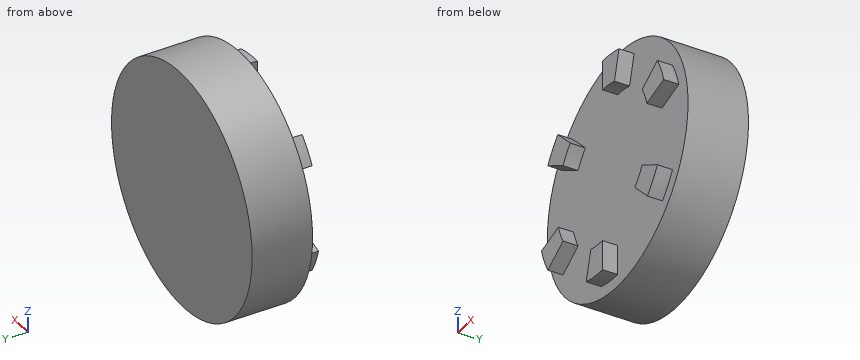
from build123d import *

# Parameters (mm, degrees)
F0_R     = 25.4
F1_DEPTH = 12.7
F2_DEPTH = 15.875


# Not quite as in the source:
# - a length typed as a fraction of an inch, garbled in the dataset ("3 / 203.2 mm" for 3/8 in), is restored
# - a feature names something its author has since deleted; it is built from what else it names


with BuildPart() as f1:
    # F0 (on Front) → F1 (new body)
    with BuildSketch(Plane.XZ):
        Circle(F0_R)
        with BuildLine():
            Line((0, -16.51), (0, -22.86))
            ThreePointArc((0, -22.86), (-2.9838287542, -22.664429531), (-5.916603371, -22.081064389))
            Line((-5.916603371, -22.081064389), (-4.2731024346, -15.947435392))
            ThreePointArc((-4.2731024346, -15.947435392), (-2.1549874336, -16.3687546613), (0, -16.51))
        make_face(mode=Mode.SUBTRACT)
        with BuildLine():
            Line((-14.2980794165, -8.255), (-19.7973407305, -11.43))
            ThreePointArc((-19.7973407305, -11.43), (-21.1198861132, -8.7481432639), (-22.081064389, -5.916603371))
            Line((-22.081064389, -5.916603371), (-15.947435392, -4.2731024346))
            ThreePointArc((-15.947435392, -4.2731024346), (-15.2532510818, -6.3181034683), (-14.2980794165, -8.255))
        make_face(mode=Mode.SUBTRACT)
        with BuildLine():
            Line((14.2980794165, -8.255), (19.7973407305, -11.43))
            ThreePointArc((19.7973407305, -11.43), (18.1360573591, -13.9162862671), (16.1644610179, -16.1644610179))
            Line((16.1644610179, -16.1644610179), (11.6743329574, -11.6743329574))
            ThreePointArc((11.6743329574, -11.6743329574), (13.0982636482, -10.0506511929), (14.2980794165, -8.255))
        make_face(mode=Mode.SUBTRACT)
        with BuildLine():
            Line((-14.2980794165, 8.255), (-19.7973407305, 11.43))
            ThreePointArc((-19.7973407305, 11.43), (-18.1360573591, 13.9162862671), (-16.1644610179, 16.1644610179))
            Line((-16.1644610179, 16.1644610179), (-11.6743329574, 11.6743329574))
            ThreePointArc((-11.6743329574, 11.6743329574), (-13.0982636482, 10.0506511929), (-14.2980794165, 8.255))
        make_face(mode=Mode.SUBTRACT)
        with BuildLine():
            Line((14.2980794165, 8.255), (19.7973407305, 11.43))
            ThreePointArc((19.7973407305, 11.43), (21.1198861132, 8.7481432639), (22.081064389, 5.916603371))
            Line((22.081064389, 5.916603371), (15.947435392, 4.2731024346))
            ThreePointArc((15.947435392, 4.2731024346), (15.2532510818, 6.3181034683), (14.2980794165, 8.255))
        make_face(mode=Mode.SUBTRACT)
        with BuildLine():
            Line((0, 16.51), (0, 22.86))
            ThreePointArc((0, 22.86), (2.9838287542, 22.664429531), (5.916603371, 22.081064389))
            Line((5.916603371, 22.081064389), (4.2731024346, 15.947435392))
            ThreePointArc((4.2731024346, 15.947435392), (2.1549874336, 16.3687546613), (0, 16.51))
        make_face(mode=Mode.SUBTRACT)
        with BuildLine():
            ThreePointArc((5.916603371, 22.081064389), (2.9838287542, 22.664429531), (0, 22.86))
            Line((0, 22.86), (0, 16.51))
            ThreePointArc((0, 16.51), (2.1549874336, 16.3687546613), (4.2731024346, 15.947435392))
            Line((4.2731024346, 15.947435392), (5.916603371, 22.081064389))
        make_face()
        with BuildLine():
            ThreePointArc((-16.1644610179, 16.1644610179), (-18.1360573591, 13.9162862671), (-19.7973407305, 11.43))
            Line((-19.7973407305, 11.43), (-14.2980794165, 8.255))
            ThreePointArc((-14.2980794165, 8.255), (-13.0982636482, 10.0506511929), (-11.6743329574, 11.6743329574))
            Line((-11.6743329574, 11.6743329574), (-16.1644610179, 16.1644610179))
        make_face()
        with BuildLine():
            ThreePointArc((-22.081064389, -5.916603371), (-21.1198861132, -8.7481432639), (-19.7973407305, -11.43))
            Line((-19.7973407305, -11.43), (-14.2980794165, -8.255))
            ThreePointArc((-14.2980794165, -8.255), (-15.2532510818, -6.3181034683), (-15.947435392, -4.2731024346))
            Line((-15.947435392, -4.2731024346), (-22.081064389, -5.916603371))
        make_face()
        with BuildLine():
            ThreePointArc((16.1644610179, -16.1644610179), (18.1360573591, -13.9162862671), (19.7973407305, -11.43))
            Line((19.7973407305, -11.43), (14.2980794165, -8.255))
            ThreePointArc((14.2980794165, -8.255), (13.0982636482, -10.0506511929), (11.6743329574, -11.6743329574))
            Line((11.6743329574, -11.6743329574), (16.1644610179, -16.1644610179))
        make_face()
        with BuildLine():
            ThreePointArc((22.081064389, 5.916603371), (21.1198861132, 8.7481432639), (19.7973407305, 11.43))
            Line((19.7973407305, 11.43), (14.2980794165, 8.255))
            ThreePointArc((14.2980794165, 8.255), (15.2532510818, 6.3181034683), (15.947435392, 4.2731024346))
            Line((15.947435392, 4.2731024346), (22.081064389, 5.916603371))
        make_face()
        with BuildLine():
            ThreePointArc((-5.916603371, -22.081064389), (-2.9838287542, -22.664429531), (0, -22.86))
            Line((0, -22.86), (0, -16.51))
            ThreePointArc((0, -16.51), (-2.1549874336, -16.3687546613), (-4.2731024346, -15.947435392))
            Line((-4.2731024346, -15.947435392), (-5.916603371, -22.081064389))
        make_face()
    extrude(amount=F1_DEPTH)

    # F0 (on Front) → F2 (join)
    with BuildSketch(Plane.XZ):
        with BuildLine():
            ThreePointArc((22.081064389, 5.916603371), (21.1198861132, 8.7481432639), (19.7973407305, 11.43))
            Line((19.7973407305, 11.43), (14.2980794165, 8.255))
            ThreePointArc((14.2980794165, 8.255), (15.2532510818, 6.3181034683), (15.947435392, 4.2731024346))
            Line((15.947435392, 4.2731024346), (22.081064389, 5.916603371))
        make_face()
        with BuildLine():
            ThreePointArc((16.1644610179, -16.1644610179), (18.1360573591, -13.9162862671), (19.7973407305, -11.43))
            Line((19.7973407305, -11.43), (14.2980794165, -8.255))
            ThreePointArc((14.2980794165, -8.255), (13.0982636482, -10.0506511929), (11.6743329574, -11.6743329574))
            Line((11.6743329574, -11.6743329574), (16.1644610179, -16.1644610179))
        make_face()
        with BuildLine():
            ThreePointArc((-5.916603371, -22.081064389), (-2.9838287542, -22.664429531), (0, -22.86))
            Line((0, -22.86), (0, -16.51))
            ThreePointArc((0, -16.51), (-2.1549874336, -16.3687546613), (-4.2731024346, -15.947435392))
            Line((-4.2731024346, -15.947435392), (-5.916603371, -22.081064389))
        make_face()
        with BuildLine():
            ThreePointArc((-16.1644610179, 16.1644610179), (-18.1360573591, 13.9162862671), (-19.7973407305, 11.43))
            Line((-19.7973407305, 11.43), (-14.2980794165, 8.255))
            ThreePointArc((-14.2980794165, 8.255), (-13.0982636482, 10.0506511929), (-11.6743329574, 11.6743329574))
            Line((-11.6743329574, 11.6743329574), (-16.1644610179, 16.1644610179))
        make_face()
        with BuildLine():
            ThreePointArc((5.916603371, 22.081064389), (2.9838287542, 22.664429531), (0, 22.86))
            Line((0, 22.86), (0, 16.51))
            ThreePointArc((0, 16.51), (2.1549874336, 16.3687546613), (4.2731024346, 15.947435392))
            Line((4.2731024346, 15.947435392), (5.916603371, 22.081064389))
        make_face()
        with BuildLine():
            ThreePointArc((-22.081064389, -5.916603371), (-21.1198861132, -8.7481432639), (-19.7973407305, -11.43))
            Line((-19.7973407305, -11.43), (-14.2980794165, -8.255))
            ThreePointArc((-14.2980794165, -8.255), (-15.2532510818, -6.3181034683), (-15.947435392, -4.2731024346))
            Line((-15.947435392, -4.2731024346), (-22.081064389, -5.916603371))
        make_face()
    extrude(amount=F2_DEPTH)


solid = f1.part
Geometry: final body of the model. Coordinates: model frame, mm. Give positions to 0.01 mm unless a question says otherwise; leave off trailing zeros. Write each loop counter-clockwise with the first axis right and the second up, starting at its lowest first coordinate (ties: lowest second). Pieces come first, ordered by that corner, then holes. Notation, with made-up numbers: M 7,3 L 41,3 A13 ccw 41,19 Z; hole C 52.5,-7.5 d10. An arc over 180 degrees is marked long. Answer in a Markdown table with one row per item. Add a question column.
(1) Section D-D on z = -9. Return loops of the section in (x, y) (3 decimals), and give its area (3 significant figures).
(2) Section C-C on z = 0. Return loops of the section in (x, y).
(3) First-contact query: pin 1 (12 mm diameter, centred on x = 12, z = 2, fed in from +Y); pin 2 (8 mm diameter, centred on x = 19, y = -1.5, fed in from -Z); pin 3 (2.5 mm diameter, centred on y = -14.5, z = -19, fed in from +X); pin 4 (8 mm diameter, centred on y = -12.5, z = -13, fed in from -X). Flat tips, straight axial feed; report the tip coordinate or a pass-through.
(4) Ray query, line 1 (Y direction, x = 0, z = -3.5); line 2 (X direction, y = -13.75, z = 8.5); line 3 (Z direction, x = 21, y = -2.75). Return the intervals inside material, ascending.
(5) Section B-B on y = -3.5. Return loops of the section in (x, z).
(6) Section A-A on z = 20.5. Return loops of the section in (x, y) (3 decimals), and give its area (3 significant figures).
Result set:
| question | item | result |
|---|---|---|
| 1 | outline | M -23.752,-12.7 L -21.014,-12.7 L -21.014,-15.875 L -15.588,-15.875 L -15.588,-12.7 L 13.841,-12.7 L 13.841,-15.875 L 15.588,-15.875 L 15.588,-12.7 L 23.752,-12.7 L 23.752,0 L -23.752,0 Z |
| 1 | area | 626 mm^2 |
| 2 | outline | M -25.4,-12.7 L 25.4,-12.7 L 25.4,0 L -25.4,0 Z |
| 3 | pin 1 | stops at y = 0 |
| 3 | pin 2 | stops at z = -20.5 |
| 3 | pin 3 | stops at x = 0 |
| 3 | pin 4 | stops at x = -23.75 |
| 4 | line 1 | y = -12.7 to 0 |
| 4 | line 2 | x = -14.72 to -14.15, 14.72 to 21.22 |
| 4 | line 3 | z = -14.29 to 14.29 |
| 5 | outline | C 0,0 d50.8 |
| 6 | outline | M -14.997,-12.7 L 0,-12.7 L 0,-15.875 L 5.493,-15.875 L 5.493,-12.7 L 14.997,-12.7 L 14.997,0 L -14.997,0 Z |
| 6 | area | 398 mm^2 |
